Input: part model. Units: mm. Frame: model coordinates. A direction names the side the tool comes from. Coordinates: 2 decimals unless noted, no trailing zeros. Loops run counter-clockwise (first coordinate to the right, second up) from the corner with the lowest first, then second, coordinate; pieces in that order, holes last. Notation, with made-up numbers: (-14, -29.75) - (34, -29.75) arc R16 cw to (34, -10.75) - close; hole circle Ø7 at (11.25, 33). An arc over 180 degrees is marked (long way). Use one line per item in the form item = value.
from build123d import *

# Parameters (mm, degrees)
FCE_00_TRIM_END_DEPTH             = 58.943741301
FCE_00_TRIM_END_DEPTH_BACK        = 58.943741301
F_5_8_11_TAPPED_HOLE1_D           = 13.49248
F_5_8_11_TAPPED_HOLE1_DEPTH       = 40.1193
F_5_8_11_TAPPED_HOLE1_CSINK_D     = 16.6624
F_5_8_11_TAPPED_HOLE1_CSINK_ANGLE = 90
F_5_8_11_TAPPED_HOLE1_TIP         = 4.053549943
FCH_00_CHAMFER_0_015_SIZE         = 0.381


with BuildPart() as part:
    # Sketch3 → FBR-00 Basic blank revolve. (revolve)
    with BuildSketch(Plane(origin=(0, 0, 0), x_dir=(0, 0, -1), z_dir=(1, 0, 0)), mode=Mode.PRIVATE) as fbr_00_basic_blank_revolve_sk:
        with BuildLine():
            Line((-45.466, 0), (-12.115698454, 0))
            Line((-12.115698454, 0), (-7.366, 19.05))
            Line((-7.366, 19.05), (8.509, 19.05))
            Line((8.509, 19.05), (8.509, 22.76475))
            ThreePointArc((8.509, 22.76475), (8.434605122, 22.944355122), (8.255, 23.01875))
            Line((8.255, 23.01875), (7.62, 23.01875))
            Line((7.62, 23.01875), (7.239, 23.1394))
            Line((7.239, 23.1394), (6.096, 23.1394))
            Line((6.096, 23.1394), (4.602815367, 21.646215367))
            ThreePointArc((4.602815367, 21.646215367), (4.064, 21.423030735), (3.525184633, 21.646215367))
            Line((3.525184633, 21.646215367), (2.032, 23.1394))
            Line((2.032, 23.1394), (0, 23.1394))
            Line((0, 23.1394), (0, 23.9014))
            Line((0, 23.9014), (-0.508, 23.9014))
            ThreePointArc((-0.508, 23.9014), (-0.799604775, 23.843396204), (-1.046815367, 23.678215367))
            Line((-1.046815367, 23.678215367), (-1.387974388, 23.337056347))
            ThreePointArc((-1.387974388, 23.337056347), (-2.451768264, 22.975946985), (-3.385852263, 23.600081959))
            Line((-3.385852263, 23.600081959), (-4.425035428, 25.4))
            Line((-4.425035428, 25.4), (-45.466, 25.4))
            Line((-45.466, 25.4), (-45.466, 0))
        make_face()
    revolve(fbr_00_basic_blank_revolve_sk.sketch.rotate(Axis((0, 0, -27.766671499), (0, 0, 1)), 90), axis=Axis((0, 0, -27.766671499), (0, 0, 1)))

    # Sketch19 → FCE-00 Trim end. (cut, two sides: drawn at the far end of the back side and taken through both)
    with BuildSketch(Plane(origin=(0, 0, 0), x_dir=(0, 0, -1), z_dir=(1, 0, 0)).offset(-FCE_00_TRIM_END_DEPTH_BACK)):
        Polygon((-68.346920588, -205.891877202), (-47.536496087, -33.923795537), (-39.26053446, 34.465066253), (-18.450109959, 206.433147918), (-362.38627329, 248.05399692), (-412.283083919, -164.271028201), align=None)
    extrude(amount=FCE_00_TRIM_END_DEPTH + FCE_00_TRIM_END_DEPTH_BACK, mode=Mode.SUBTRACT)

    # 5/8-11 Tapped Hole1
    with Locations(Plane(origin=(0, 2.097889548, 43.17739322), x_dir=(0, 0.992757341929, -0.120136838835), z_dir=(0, 0.120136838835, 0.992757341929))):
        with Locations((0, 0)):
            CounterSinkHole(F_5_8_11_TAPPED_HOLE1_D / 2, F_5_8_11_TAPPED_HOLE1_CSINK_D / 2, depth=F_5_8_11_TAPPED_HOLE1_DEPTH, counter_sink_angle=F_5_8_11_TAPPED_HOLE1_CSINK_ANGLE)
            with Locations((0, 0, -(F_5_8_11_TAPPED_HOLE1_DEPTH + F_5_8_11_TAPPED_HOLE1_TIP / 2))):  # 118° drill point
                Cone(0, F_5_8_11_TAPPED_HOLE1_D / 2, F_5_8_11_TAPPED_HOLE1_TIP, mode=Mode.SUBTRACT)

    # FCS-00 Bevel.: sweep along a path in Sketch22
    with BuildLine(Plane(origin=(0, -16.814137816, 45.466), x_dir=(-1, 0, 0), z_dir=(0, -0.11996356816283467, -0.9927782946426865))) as fcs_00_bevel_path:
        Line((-3.175, 0.403277876), (3.175, 0.403277876))
        ThreePointArc((3.175, 0.403277876), (3.975127257, 0.453889304), (4.7625, 0.604916814))
        ThreePointArc((4.7625, 0.604916814), (0, 38.1), (-4.7625, 0.604916814))
        ThreePointArc((-4.7625, 0.604916814), (-3.975127257, 0.453889304), (-3.175, 0.403277876))
    # Sketch31 → FCS-00 Bevel. (sweep, cut)
    with BuildSketch(Plane(origin=(0, 0, 0), x_dir=(0, 0, -1), z_dir=(1, 0, 0))):
        Polygon((-46.883705055, -15.313405584), (-11.697696067, -41.722206608), (-12.459464725, -48.026348779), (-50.284317751, -43.455736832), align=None)
    sweep(path=fcs_00_bevel_path.line, mode=Mode.SUBTRACT)

    # FCH-00 Chamfer 0.015
    fch_00_chamfer_0_015_edges = [part.edges().sort_by_distance(p)[0] for p in [
        (19.05, 0, -8.509),
    ]]
    chamfer(fch_00_chamfer_0_015_edges, length=FCH_00_CHAMFER_0_015_SIZE)


solid = part.part
Q1. Cut plane A-A, the plane z = -1. Return loops of the section in (x, y).
Check values:
outline = circle Ø46.28 at (0, 0); hole circle Ø38.1 at (0, 0)
Q2. First-contact query: P1, Ø5, axis at y = -7, z = 20.5, coming from the +X side; P2, Ø8, axis at x = 2.5, z = -1, coming from the +Y side; P3, Ø10, axis at x = -6.5, y = -8.5, coming from the -Z side. Flat tips, straight axial feed; report the tip coordinate or a pass-through.
Check values:
P1 = 25
P2 = 23.9
P3 = 8.2
Q3. Ray query, line 1 along Y through (x, z) = (0, 0.25); line 2 along Y through (x, z) = (0, -1.5); line 3 along X through (y, z) = (0.5, 7). Return the intervals inside material, ascending. Write a range as [from, to].
Check values:
line_1 = [-23.9, -19.05], [19.05, 23.9]
line_2 = [-23.14, -19.05], [19.05, 23.14]
line_3 = [-25.4, -19.04], [19.04, 25.4]
Q4. Pull-direction query (X, two-part tool) for faces 1 (the conical face through (-2.706, 5.202, 10.654)), 2 (the flat face through (17, -10, -8.509)), 3 (the conical face through (6.1, -1.2, 42.1)), 4 (the cylindrical face through (4.99, 22.47, -7.93)); classes: pulls with the +X half, pulls with the -X half, needs draft (parallel to the pull), parting line crosses it, or undercut.
Check values:
face_1 = undercut
face_2 = needs draft
face_3 = undercut
face_4 = parting line crosses it
Q5. Set-up query: faces 5 (the cylindrical face through (-2.026, -6.473, 25.913)), 6 (the cylindrical face through (3.012, -22.942, -6.659)). Return all of +Z, -Z, +X, -X, +Y, -Y with unobstructed straight access to the full face (end or side cutting, diameter ignored); none if empty.
Check values:
face_5 = none
face_6 = -Z
